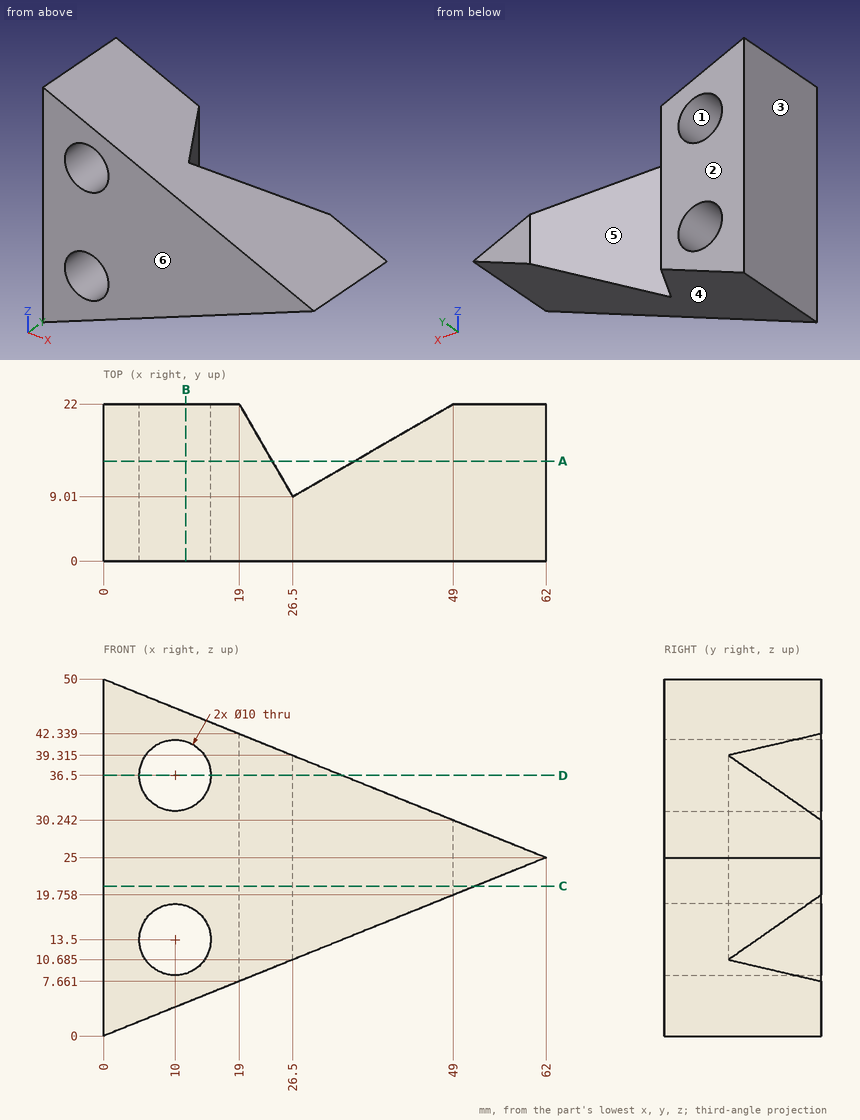
For this review, use the dimensioned drawing (mm, ordinates from the lowest corner) and the shaded views. A direction names the side the tool comes from. Round coordinates to 2 decimals unless told otherwise and drop trailing zeros. Order: outer loops, then holes, each group sorted by start corner. A loop starts at its lowest first (then second) coordinate and runs counter-clockwise, first axis right, second up. Notation, with made-up numbers: (11, 57) - (28, 57) arc R24 cw to (28, 87) - close; hole circle Ø4 at (-23, -1.75). An arc over 180 degrees is marked (long way). Use one line per item in the form item = value.
Q1. To check wall thickness, follow line 1 (X direction, y = 12.25, z = 36.5) (1 decimal); line 2 (Z direction, x = 14, y = 19.5) (1 decimal); line 3 (X direction, y = 9.25, z = 13.5) (1 decimal). State the ranges of each line that lie inside material, in increasing order.
Response values:
line_1 = 0 to 5, 15 to 24.6, 32.1 to 33.5
line_2 = 5.6 to 10.5, 16.5 to 33.5, 39.5 to 44.4
line_3 = 0 to 5, 15 to 26.4, 26.9 to 33.5
Q2. Clearance check with flat-ended pins moving along their axes: P1, Ø12, axis at y = 19.5, z = 6.5, coming from the -X side; P2, Ø8, axis at x = 45, z = 32.5, coming from the +Y side; P3, Ø3, axis at x = 52, y = 15, coming from the +Z side; P4, Ø2, axis at x = 49, z = 17.5, coming from the +Y side. State where each tip first meets the part, or that it passes through.
Response values:
P1 = 0
P2 = 21.68
P3 = 29.64
P4 = through
Q3. Add section C-C on z = 21. Give the boundary of the cut face in (x, y), then the cut area to 3 significant figures.
Response values:
outline = (0, 0) - (52.08, 0) - (52.08, 22) - (49, 22) - (26.5, 9.01) - (19, 22) - (0, 22) - close
area = 951 mm^2
Q4. Add section A-A on y = 14. Give the boundary of the cut face in (x, z).
Response values:
outline = (0, 0) - (23.62, 9.52) - (23.62, 40.48) - (0, 50) - close; (35.14, 14.17) - (62, 25) - (35.14, 35.83) - close; hole circle Ø10 at (10, 13.5); hole circle Ø10 at (10, 36.5)
Q5. Mouldability with a two-part tool opening along X and no side actions: class the marked faces 1, 2, 3 and 4 as pulls with the +X half, pulls with the -X half, needs draft (parallel to the pull), parting line crosses it, or undercut.
Response values:
face_1 = undercut
face_2 = needs draft
face_3 = pulls with the -X half
face_4 = pulls with the +X half
Q6. Add section D-D on z = 36.5. Give the boundary of the cut face in (x, y), then the cut area to 3 significant figures.
Response values:
outline = (0, 0) - (5, 0) - (5, 22) - (0, 22) - close; (15, 0) - (33.48, 0) - (33.48, 13.04) - (26.5, 9.01) - (19, 22) - (15, 22) - close
area = 391 mm^2
Q7. Tool access review of the marked faces 5 and 6: name each direction out of +Z, -Z, +X, -X, +Y, -Y from which nothing blocks a thin tool from reaching the whole face with its end or side.
Response values:
face_5 = +Z, -Z, +Y
face_6 = +Z, -Z, +X, -X, -Y
Q8. Add section B-B on x = 11.5. Give the boundary of the cut face in (y, z), then the cut area to 3 significant figures.
Response values:
outline = (0, 4.64) - (22, 4.64) - (22, 8.73) - (0, 8.73) - close; (0, 18.27) - (22, 18.27) - (22, 31.73) - (0, 31.73) - close; (0, 41.27) - (22, 41.27) - (22, 45.36) - (0, 45.36) - close
area = 476 mm^2
